Verification items for the finished model (mm, model axes). Face numbers are marked on the shaded views. A direction names the side the tool comes from. Round coordinates to 2 decimals unless told otherwise and drop trailing zeros. Order: outer loops, then holes, each group sorted by start corner. A loop starts at its lowest first (then second) coordinate and runs counter-clockwise, first axis right, second up. Notation, with made-up numbers: (13.5, 9.25) -> (59.5, 9.25) arc R7 ccw to (59.5, 19.25) -> close; hole circle Ø1 at (78, -8). An arc over 180 degrees is marked (long way). Return JSON: item names as keys, results as strings. Group by question number.
1) Scan lines: L1, parallel to Y at x = 10.75, z = -12; L2, parallel to Y at x = -5.75, z = -8.25; L3, parallel to Z at x = -2, y = 1. Record each from-to range of solid material in increasing order.
2) Section check B-B on z = -6.75. Enter the section's corners in (x, y), plus the area to 3 significant figures.
3) Tool access check on the marked faces 1, 2, 3 and 4. Record the directions out of +Z, -Z, +X, -X, +Y, -Y that give a thin tool (end or side, any length) a straight path to the whole face; none if there is none.
4) Section check A-A on x = 0. Enter the section's corners in (y, z).
5) Depth check by flat-ended pin: pin 1 (3.5 mm diameter, centred on x = -0.5, y = 4, fed in from -Z). Enter the tip coordinate at first touch or a pass-through.
6) Draft check along Y on the marked faces 5, 6, 7 and 8. Enter one of: pulls with the +Y half, pulls with the -Y half, needs draft (parallel to the pull), parting line crosses it, or undercut.
7) Section check C-C on y = 9.25. Enter the section's corners in (x, z).
8) Section check D-D on z = 5.5. Enter the section's corners in (x, y), plus the area to 3 significant figures.
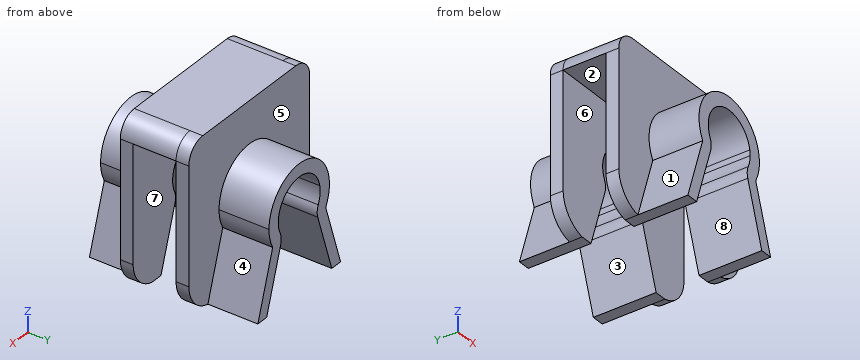
```python
from build123d import *

# Parameters (mm, degrees)
F1_DEPTH = 9.8
F2_DEPTH = 2
F3_R     = 3
F5_DEPTH = 3.35
F7_R     = 2.5


with BuildPart() as f1:
    # F0 (on Front) → F1 (new body)
    with BuildSketch(Plane.XZ):
        with BuildLine():
            ThreePointArc((6.5, 0), (-1.6120548351, 6.2969261714), (-5.7003936026, -3.1233816249))
            Line((-5.7003936026, -3.1233816249), (-4.4224832798, 0.8316499504))
            ThreePointArc((-4.4224832798, 0.8316499504), (0, 4.5), (4.4224832798, 0.8316499504))
            Line((4.4224832798, 0.8316499504), (5.7003936026, -3.1233816249))
            ThreePointArc((5.7003936026, -3.1233816249), (6.2969261714, -1.6120548351), (6.5, 0))
        make_face()
        with BuildLine():
            Line((-4.4224832798, 0.8316499504), (-5.7003936026, -3.1233816249))
            ThreePointArc((-5.7003936026, -3.1233816249), (-5.1003989607, -4.0293833824), (-4.3578547765, -4.8227690953))
            Line((-4.3578547765, -4.8227690953), (-3.65, -2.6320144377))
            ThreePointArc((-3.65, -2.6320144377), (-4.3920939566, -0.9795461582), (-4.4224832798, 0.8316499504))
        make_face()
        with BuildLine():
            Line((-5.7003936026, -3.1233816249), (-8.891627942, -13))
            Line((-8.891627942, -13), (-7, -13))
            Line((-7, -13), (-4.3578547765, -4.8227690953))
            ThreePointArc((-4.3578547765, -4.8227690953), (-5.1003989607, -4.0293833824), (-5.7003936026, -3.1233816249))
        make_face()
        with BuildLine():
            Line((7, -13), (8.891627942, -13))
            Line((8.891627942, -13), (5.7003936026, -3.1233816249))
            ThreePointArc((5.7003936026, -3.1233816249), (5.1003989607, -4.0293833824), (4.3578547765, -4.8227690953))
            Line((4.3578547765, -4.8227690953), (7, -13))
        make_face()
        with BuildLine():
            ThreePointArc((4.3578547765, -4.8227690953), (5.1003989607, -4.0293833824), (5.7003936026, -3.1233816249))
            Line((5.7003936026, -3.1233816249), (4.4224832798, 0.8316499504))
            ThreePointArc((4.4224832798, 0.8316499504), (4.4805789112, 0.4176273704), (4.5, 0))
            ThreePointArc((4.5, 0), (4.2822307271, -1.3829316686), (3.65, -2.6320144377))
            Line((3.65, -2.6320144377), (4.3578547765, -4.8227690953))
        make_face()
    extrude(amount=F1_DEPTH)

    # F0 (on Front) → F2 (join)
    with BuildSketch(Plane.XZ):
        with BuildLine():
            Line((13, 13), (-13, 13))
            Line((-13, 13), (-13, -8.2140415907))
            ThreePointArc((-13, -8.2140415907), (-11.7956860143, -11.3365696666), (-8.891627942, -13))
            Line((-8.891627942, -13), (-5.7003936026, -3.1233816249))
            ThreePointArc((-5.7003936026, -3.1233816249), (-1.6120548351, 6.2969261714), (6.5, 0))
            ThreePointArc((6.5, 0), (6.2969261714, -1.6120548351), (5.7003936026, -3.1233816249))
            Line((5.7003936026, -3.1233816249), (8.891627942, -13))
            ThreePointArc((8.891627942, -13), (11.7956860143, -11.3365696666), (13, -8.2140415907))
            Line((13, -8.2140415907), (13, 13))
        make_face()
    extrude(amount=F2_DEPTH)

    # F3
    f3_edges = [f1.edges().sort_by_distance(p)[0] for p in [
        (-13, -1, 13),
        (13, -1, 13),
    ]]
    fillet(f3_edges, radius=F3_R)

    # F4 (on face) → F5 (join)
    with BuildSketch(Plane.XZ):
        with BuildLine():
            ThreePointArc((13, 10), (12.1213203436, 12.1213203436), (10, 13))
            Line((10, 13), (-10, 13))
            ThreePointArc((-10, 13), (-12.1213203436, 12.1213203436), (-13, 10))
            Line((-13, 10), (13, 10))
        make_face()
    extrude(amount=-F5_DEPTH)

    # F6: F1 across face


with BuildPart() as f1_1:
    add(f1.part)
    add(f1.part.mirror(Plane(origin=(0, 3.35, 11.4567592), x_dir=(1, 0, 0), z_dir=(0, 1, 0))))

    # F7
    f7_edges = [f1_1.edges().sort_by_distance(p)[0] for p in [
        (-3.65, -4.9, -2.632014),
        (-3.65, 11.6, -2.632014),
        (3.65, 11.6, -2.632014),
        (3.65, -4.9, -2.632014),
    ]]
    fillet(f7_edges, radius=F7_R)


solid = f1_1.part
```
Check result:
{
 "1": {"L1": "-2 to 0, 6.7 to 8.7", "L2": "-9.8 to 0, 6.7 to 16.5", "L3": "10 to 13"},
 "2": {"outline": "(-13, -2) -> (-6.87, -2) -> (-6.87, -9.8) -> (-4.98, -9.8) -> (-4.98, 0) -> (-13, 0) -> close; (-13, 6.7) -> (-4.98, 6.7) -> (-4.98, 16.5) -> (-6.87, 16.5) -> (-6.87, 8.7) -> (-13, 8.7) -> close; (4.98, -9.8) -> (6.87, -9.8) -> (6.87, -2) -> (13, -2) -> (13, 0) -> (4.98, 0) -> close; (4.98, 6.7) -> (13, 6.7) -> (13, 8.7) -> (6.87, 8.7) -> (6.87, 16.5) -> (4.98, 16.5) -> close", "area": "123 mm^2"},
 "3": {"face 1": "-X, -Y", "face 2": "-Z, +X, -X", "face 3": "-Z, +Y, -Y", "face 4": "+X, +Y"},
 "4": {"outline": "(-9.8, 4.5) -> (0, 4.5) -> (0, 10) -> (6.7, 10) -> (6.7, 4.5) -> (16.5, 4.5) -> (16.5, 6.5) -> (8.7, 6.5) -> (8.7, 13) -> (-2, 13) -> (-2, 6.5) -> (-9.8, 6.5) -> close"},
 "5": {"pin 1": "z = 10"},
 "6": {"face 5": "pulls with the +Y half", "face 6": "undercut", "face 7": "undercut", "face 8": "needs draft"},
 "7": {"outline": "(-8.89, -13) -> (-7, -13) -> (-3.99, -3.68) arc R2.5 ccw to (-4.09, -1.87) arc R4.5 cw (long way) to (4.09, -1.87) arc R2.5 ccw to (3.99, -3.68) -> (7, -13) -> (8.89, -13) -> (5.7, -3.12) arc R6.5 ccw (long way) to (-5.7, -3.12) -> close"},
 "8": {"outline": "(-13, -2) -> (-3.46, -2) -> (-3.46, -9.8) -> (3.46, -9.8) -> (3.46, -2) -> (13, -2) -> (13, 0) -> (-13, 0) -> close; (-13, 6.7) -> (13, 6.7) -> (13, 8.7) -> (3.46, 8.7) -> (3.46, 16.5) -> (-3.46, 16.5) -> (-3.46, 8.7) -> (-13, 8.7) -> close", "area": "212 mm^2"}
}
